Geometry: see drawing. Coordinates: mm, zero at the bounding-box minimum. A direction names the side the tool comes from. Give positions to 0.01 mm unless a question says otherwise; leave off trailing zeros. Write each loop counter-clockwise with the first axis right and the second up, starting at its lowest first coordinate (ties: lowest second). Pieces come first, ordered by that corner, then holes. Notation, with made-up numbers: (64.25, -28.75) - (83.25, -28.75) arc R28 ccw to (83.25, 9.25) - close; hole circle Ø5 at (57, 87.25). An arc over 180 degrees is marked (long way). Answer as CSV lines item,"result". Start each with the question number.
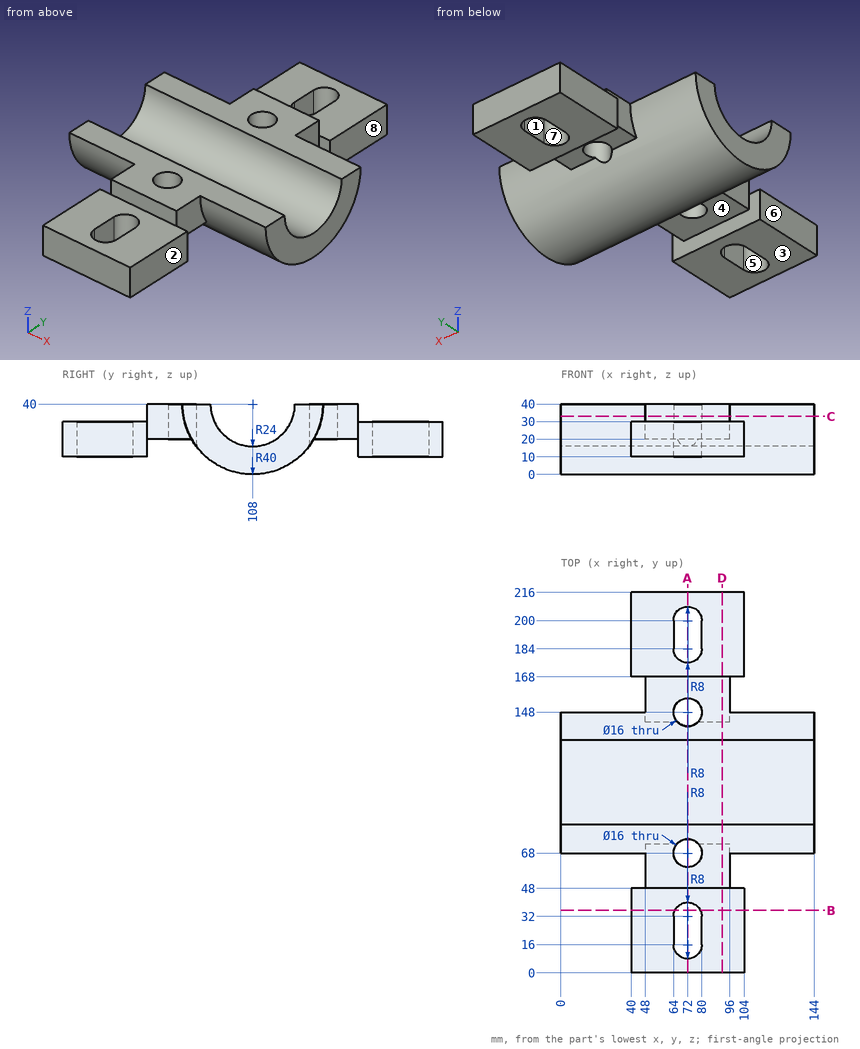
1) Pull-direction query (X, two-part tool) for the marked faces 5, 6, 7 and 8; classes: +X half, -X half, draft (parallel to the pull), parting line (faces both ways), or undercut.
2) Reachability of the marked faces 1, 2, 3 and 4 from +Z, -Z, +X, -X, +Y, -Y: full face, straight path, thin tool, end or side. Return the list, or none.
3) Cut plane D-D on x = 91.5. Output: boundary loops of the cut face in (y, z).
4) Cut plane A-A on x = 72. State how many separate pieces and enclosed holes the cut face has, and give its area (3 significant figures).
5) Cut plane C-C on z = 33. Output: boundary loops of the cut face in (x, y).
6) Material intervals for line 1 (X direction, y = 148, z = 26.25); line 2 (Y direction, x = 72, z = 28.5); line 3 (Y direction, x = 43, z = 26), sorted ascending. Write a range as from..to.
7) Cut plane B-B on y = 35.5. Output: boundary loops of the cut face in (x, z), and give its area (3 significant figures).
8) Contact query for flat-ended pins moving along their axis: P1, Ø10, axis at y = 158.5, z = 26, coming from the +X side; P2, Ø5, axis at x = 38, y = 93, coming from the -Z side; P3, Ø1.5, axis at y = 50.5, z = 30.5, coming from the -X side; P4, Ø10, axis at y = 180, z = 4, coming from the -X side. Output: stop coordinate, or through.
Numbers:
1,face 5,"undercut"
1,face 6,"-X half"
1,face 7,"undercut"
1,face 8,"+X half"
2,face 1,"+Z, -Z"
2,face 2,"+Z, -Z, +X, -Y"
2,face 3,"-Z, +X, -X, -Y"
2,face 4,"-Z, +X, -X"
3,outline,"(0, 10) - (48, 10) - (48, 20) - (73.36, 20) arc R40 ccw to (142.64, 20) - (168, 20) - (168, 10) - (216, 10) - (216, 30) - (168, 30) - (168, 40) - (132, 40) arc R24 cw to (84, 40) - (48, 40) - (48, 30) - (0, 30) - close"
4,separate pieces,"5"
4,enclosed holes,"0"
4,area,"2,470 mm²"
5,outline,"(0, 68.62) - (48, 68.62) - (48, 48) - (96, 48) - (96, 68.62) - (144, 68.62) - (144, 85.04) - (0, 85.04) - close; (0, 130.96) - (144, 130.96) - (144, 147.38) - (96, 147.38) - (96, 168) - (48, 168) - (48, 147.38) - (0, 147.38) - close; hole circle Ø16 at (72, 68); hole circle Ø16 at (72, 148)"
6,line 1,"x = 48..64, 80..96"
6,line 2,"y = 0..8, 40..60, 76..86.93, 129.07..140, 156..176, 208..216"
6,line 3,"y = 0..48, 70.53..88.51, 127.49..145.47, 168..216"
7,outline,"(40, 10) - (64.81, 10) - (64.81, 30) - (40, 30) - close; (79.19, 10) - (104, 10) - (104, 30) - (79.19, 30) - close"
7,area,"992 mm²"
8,P1,"stops at x = 96"
8,P2,"stops at z = 2"
8,P3,"stops at x = 48"
8,P4,"passes through"
